from build123d import *

# Parameters (mm, degrees)
SKETCH1_R           = 5
BOSS_EXTRUDE1_DEPTH = 2
BOSS_EXTRUDE2_DEPTH = 2


with BuildPart() as part:
    # Sketch1 → Boss-Extrude1 (new body)
    with BuildSketch(Plane.XY):
        with BuildLine():
            Line((-1.5, 6.837397166), (-1.5, 26))
            Line((-1.5, 26), (1.5, 26))
            Line((1.5, 26), (1.5, 6.837397166))
            ThreePointArc((1.5, 6.837397166), (0, -7), (-1.5, 6.837397166))
        make_face()
        Circle(SKETCH1_R, mode=Mode.SUBTRACT)
    extrude(amount=BOSS_EXTRUDE1_DEPTH)

    # Sketch2 → Boss-Extrude2 (add)
    with BuildSketch(Plane(origin=(0, 0, 0), x_dir=(-1, 0, 0), z_dir=(0, 0, -1))):
        with BuildLine():
            add(Edge.make_bspline(
                [(-5.599278763, 4.200961478), (-15.258011941, -5.628125959), (0, -7)],
                knots=[0, 0, 0, 1, 1, 1], degree=2))
            add(Edge.make_bspline(
                [(-5.599278763, 4.200961478), (-7.981604162, -4.535813919), (0, -7)],
                knots=[0, 0, 0, 1, 1, 1], degree=2))
        make_face()
        with BuildLine():
            add(Edge.make_bspline(
                [(3.393610887, 6.122369243), (18.668225354, 0.049737096), (1.677508496, -6.796025695)],
                knots=[0, 0, 0, 1, 1, 1], degree=2))
            add(Edge.make_bspline(
                [(3.393610887, 6.122369243), (10.124192035, -1.414312589), (1.677508496, -6.796025695)],
                knots=[0, 0, 0, 1, 1, 1], degree=2))
        make_face()
    extrude(amount=-BOSS_EXTRUDE2_DEPTH)


solid = part.part
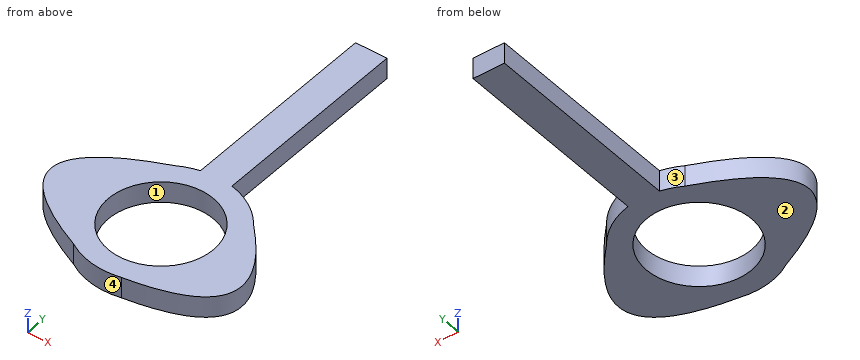
Work out the finished part from the listing and answer in its coordinate system (mm). Face numbers are marked on the shaded views. Coordinates: 2 decimals unless noted, no trailing zeros. Write each loop counter-clockwise with the first axis right and the second up, starting at its lowest first coordinate (ties: lowest second). Pieces come first, ordered by that corner, then holes.
1. Consider line 1 along Y through (x, z) = (0, 0.7); line 2 along X through (y, z) = (9.5, 0.55); line 3 along X through (y, z) = (2.5, 0.25). Determine where each line is inside the solid, lowest interval first.
Results list:
line 1: y = -7 to -5, 5 to 26
line 2: x = -1.5 to 1.5
line 3: x = -9.57 to -4.33, 4.33 to 7.14
2. The part is cut by section B-B, the plane y = 20. Write down the section's boundary in (x, z).
Results list:
outline: (-1.5, 0) - (1.5, 0) - (1.5, 2) - (-1.5, 2) - close
3. For a pull along X with two mould halves and no side action, classify the marked faces 1, 2, 3 and 4 as +X half, -X half, draft (parallel to the pull), parting line (faces both ways), or undercut.
Results list:
face 1: undercut
face 2: draft
face 3: -X half
face 4: parting line
4. Flat-ended cylindrical pins translate along their axes: pin 1 (8 mm diameter, centred on x = 0, y = 0, fed in from -Z); pin 2 (0.6 mm diameter, centred on y = 17, z = 1, fed in from +X). Find the tip coordinate at first contact, or state that the pin passes through.
Results list:
pin 1: passes through
pin 2: stops at x = 1.5
5. The part is cut by section A-A, the plane x = 0. Write down the section's boundary in (y, z), and give its area (3 significant figures).
Results list:
outline: (-7, 0) - (-5, 0) - (-5, 2) - (-7, 2) - close; (5, 0) - (26, 0) - (26, 2) - (5, 2) - close
area: 46.0 mm2
